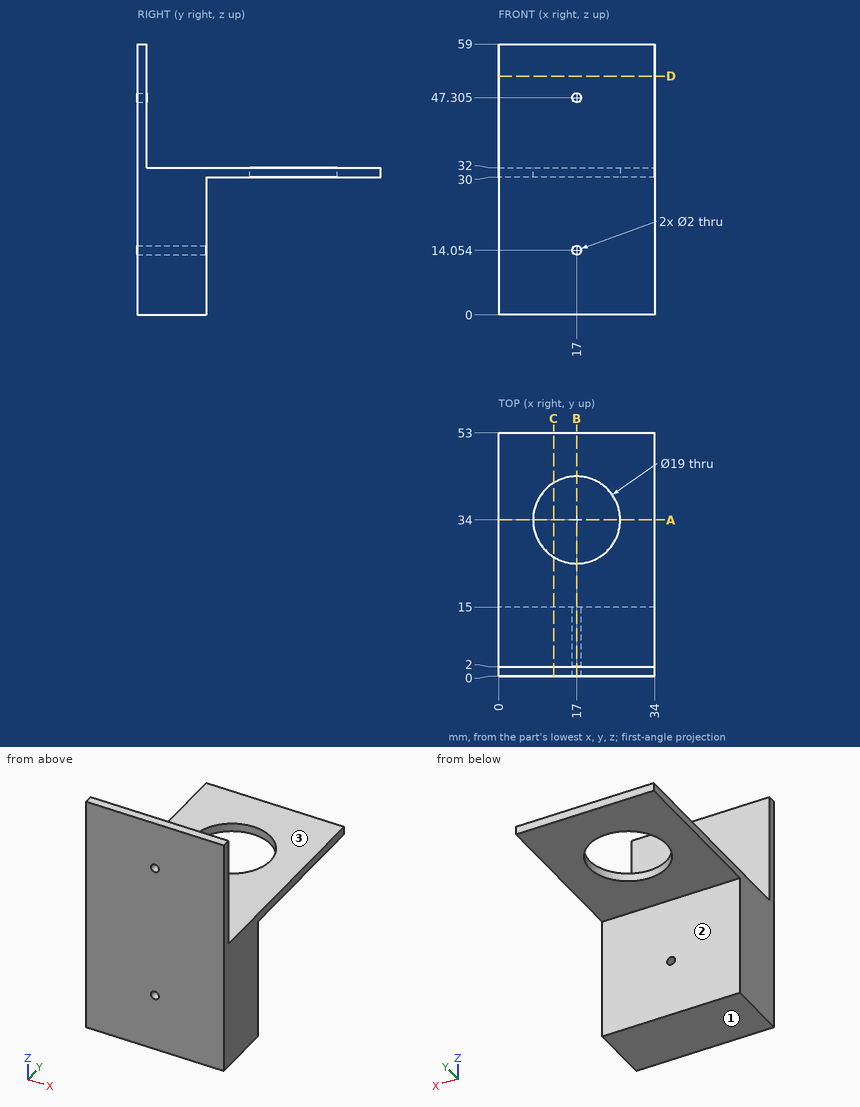
Here's the drawing with two shaded views (mm, measured from the low corner). I have some questions. A direction names the side the tool comes from. Coordinates: 2 decimals unless noted, no trailing zeros. Write each loop counter-clockwise with the first axis right and the second up, starting at its lowest first coordinate (ties: lowest second). Pieces come first, ordered by that corner, then holes.
Item 1: I want a section at B-B on x = 17. Write out the boundary of the cut face in (y, z) (1 decimal).
Item 2: I want a section at C-C on x = 12. Write out the boundary of the cut face in (y, z).
Item 3: If I drill on line 1 (Z direction, x = 17, y = 1.15) (1 decimal); line 2 (Z direction, x = 17, y = 9) (1 decimal); line 3 (Z direction, x = 6.5, y = 42), over which ranges is the centre line in solid material (lowest first)?
Item 4: I want a section at A-A on y = 34. Write out the boundary of the cut face in (x, z).
Item 5: I want a section at D-D on z = 52. Write out the boundary of the cut face in (x, y).
Item 6: Will these pins go through, and if not, where does the flat tip stop? pin 1 (17 mm diameter, centred on x = 18.5, y = 21.5, fed in from +Z); pin 2 (9 mm diameter, centred on x = 13, z = 10, fed in from +Y); pin 3 (10 mm diameter, centred on x = 26, z = 38, fed in from +Y).
Item 7: On a 3-axis mill with a long thin cutter (end or side, diameter ignored), from which of +Z, -Z, +X, -X, +Y, -Y can I reach the whole of each face in a straight line? I mean the marked faces 1, 2 and 3. Say none if no direction works.
Findings below:
1. outline: (0, 0) - (15, 0) - (15, 13.1) - (0, 13.1) - close; (0, 15.1) - (15, 15.1) - (15, 30) - (24.5, 30) - (24.5, 32) - (2, 32) - (2, 46.3) - (0, 46.3) - close; (0, 48.3) - (2, 48.3) - (2, 59) - (0, 59) - close; (43.5, 30) - (53, 30) - (53, 32) - (43.5, 32) - close
2. outline: (0, 0) - (15, 0) - (15, 30) - (25.92, 30) - (25.92, 32) - (2, 32) - (2, 59) - (0, 59) - close; (42.08, 30) - (53, 30) - (53, 32) - (42.08, 32) - close
3. line 1: z = 0 to 13.1, 15.1 to 46.3, 48.3 to 59
3. line 2: z = 0 to 13.1, 15.1 to 32
3. line 3: z = 30 to 32
4. outline: (0, 30) - (7.5, 30) - (7.5, 32) - (0, 32) - close; (26.5, 30) - (34, 30) - (34, 32) - (26.5, 32) - close
5. outline: (0, 0) - (34, 0) - (34, 2) - (0, 2) - close
6. pin 1: stops at z = 32
6. pin 2: stops at y = 15
6. pin 3: stops at y = 2
7. face 1: -Z, +X, -X, +Y, -Y
7. face 2: -Z, +X, -X, +Y
7. face 3: +Z, +X, -X, +Y
